```python
from build123d import *

# Parameters (mm, degrees)
SKETCH1_W                = 16
SKETCH1_H                = 24
SKETCH1_R                = 2.25
BOSS_EXTRUDE1_DEPTH      = 5
BOSS_EXTRUDE2_DEPTH      = 17
BOSS_EXTRUDE2_DEPTH_BACK = 5
SKETCH2_W                = 4
SKETCH2_H                = 24
SKETCH3_R                = 3.75
CUT_EXTRUDE1_DEPTH       = 30.732137495
BOSS_EXTRUDE3_DEPTH      = 2
FILLET1_R                = 3
SKETCH5_R                = 4
CUT_EXTRUDE2_DEPTH       = 2


with BuildPart() as part:
    # Sketch1 → Boss-Extrude1 (new body)
    with BuildSketch(Plane.XY):
        Rectangle(SKETCH1_W, SKETCH1_H)
        with Locations((-2, 6)):
            Circle(SKETCH1_R, mode=Mode.SUBTRACT)
        with Locations((-2, -6)):
            Circle(SKETCH1_R, mode=Mode.SUBTRACT)
    extrude(amount=BOSS_EXTRUDE1_DEPTH)

    # Sketch2 → Boss-Extrude2 (add, two sides: drawn at the far end of the back side and taken through both)
    with BuildSketch(Plane.XY.offset(5).offset(-BOSS_EXTRUDE2_DEPTH_BACK)):
        with Locations((6, 0)):
            Rectangle(SKETCH2_W, SKETCH2_H)
    extrude(amount=BOSS_EXTRUDE2_DEPTH + BOSS_EXTRUDE2_DEPTH_BACK)

    # Sketch3 → Cut-Extrude1 (cut, through all)
    with BuildSketch(Plane(origin=(8, 0, 0), x_dir=(0, 0, -1), z_dir=(1, 0, 0))):
        with Locations(Location((-14, 0, 0), (0, 0, 90))):
            Circle(SKETCH3_R)
    extrude(amount=-CUT_EXTRUDE1_DEPTH, mode=Mode.SUBTRACT)

    # Sketch4 → Boss-Extrude3 (add)
    with BuildSketch(Plane.XZ.offset(12)):
        Polygon((4, 22), (-8, 5), (4, 5), align=None)
    extrude(amount=-BOSS_EXTRUDE3_DEPTH)

    # Fillet1
    # the kernel refuses this fillet: 3 mm, written as the material it takes off along each edge
    with BuildSketch(Plane(origin=(15.5, -12, 22), x_dir=(0, 1, 0), z_dir=(-1, 0, 0))) as fillet1_piece_1:
        with BuildLine():
            CenterArc((FILLET1_R, FILLET1_R), FILLET1_R, 180, 90)
            Line((0, FILLET1_R), (0, 0))
            Line((0, 0), (FILLET1_R, 0))
        make_face()
    extrude(amount=19, mode=Mode.SUBTRACT)
    with BuildSketch(Plane(origin=(-3.5, 12, 22), x_dir=(0, 0, -1), z_dir=(1, 0, 0))) as fillet1_piece_2:
        with BuildLine():
            CenterArc((FILLET1_R, -FILLET1_R), FILLET1_R, 90, 90)
            Line((0, -FILLET1_R), (0, 0))
            Line((0, 0), (FILLET1_R, 0))
        make_face()
    extrude(amount=19, mode=Mode.SUBTRACT)
    with BuildSketch(Plane(origin=(15.5, -12, 0), x_dir=(0, 1, 0), z_dir=(-1, 0, 0)), Plane(origin=(15.5, 12, 0), x_dir=(0, 0, 1), z_dir=(-1, 0, 0))) as fillet1_piece_3:
        with BuildLine():
            CenterArc((FILLET1_R, -FILLET1_R), FILLET1_R, 90, 90)
            Line((0, -FILLET1_R), (0, 0))
            Line((0, 0), (FILLET1_R, 0))
        make_face()
    extrude(amount=31, mode=Mode.SUBTRACT)

    # Sketch5 → Cut-Extrude2 (cut)
    with BuildSketch(Plane.XY.offset(5)):
        with Locations((-2, 6)):
            Circle(SKETCH5_R)
        with Locations((-2, -6)):
            Circle(SKETCH5_R)
    extrude(amount=-CUT_EXTRUDE2_DEPTH, mode=Mode.SUBTRACT)


solid = part.part
```
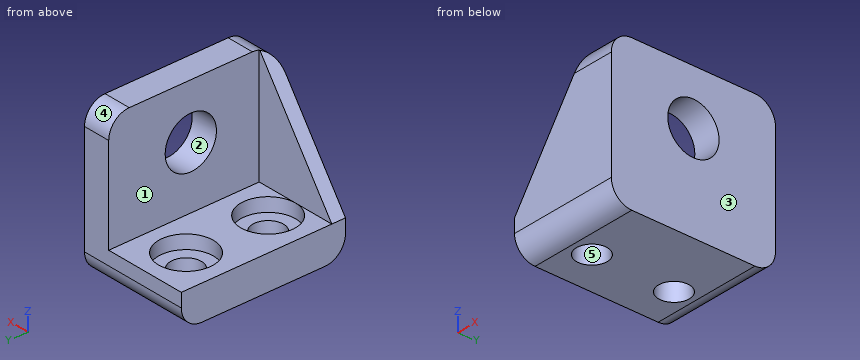
Geometry: final body of the model. Coordinates: model frame, mm. Face numbers are marked on the shaded views. A direction names the side the tool comes from. Coordinates: 2 decimals unless noted, no trailing zeros. Loops run counter-clockwise (first coordinate to the right, second up) from the corner with the lowest first, then second, coordinate; pieces in that order, holes last. Notation, with made-up numbers: M 42.25,52.5 L 71.25,52.5 A17 cw 71.25,60.5 Z; hole C 48.25,13 d8. An arc over 180 degrees is marked long. Put each result on its own line as item: value.
(1) Cut plane B-B on x = 5.75. Return the cut outline in (y, z).
Answer sheet:
outline: M -12,3 A3 ccw -9,0 L 9,0 A3 ccw 12,3 L 12,19 A3 ccw 9,22 L -9,22 A3 ccw -12,19 Z; hole C 0,14 d7.5
(2) First-contact query: pin 1 (4 mm diameter, centred on x = -3, y = -6.5, fed in from +Z); pin 2 (5 mm diameter, centred on x = -2.5, z = 16, fed in from +Y); pin 3 (10 mm diameter, centred on y = 0, z = 14, fed in from -X); pin 4 (1.5 mm diameter, centred on y = -1.5, z = 14.5, fed in from -X). Flat tips, straight axial feed; report the tip coordinate or a pass-through.
Answer sheet:
pin 1: stops at z = 3
pin 2: stops at y = -10
pin 3: stops at x = 4
pin 4: passes through
(3) Cut plane C-C on z = 12.75. Return the cut outline in (x, y), then the cut area to 3 significant figures.
Answer sheet:
outline: M -2.53,-12 L 8,-12 L 8,-3.54 L 4,-3.54 L 4,-10 L -2.53,-10 Z; M 4,3.54 L 8,3.54 L 8,12 L 4,12 Z
area: 80.8 mm^2
(4) Material intervals for probe 1 along Y at (x, z) = (-2, 4.45); probe 2 along X at (y, z) = (6, 1.15); probe 3 along Y at (x, z) = (-2, 2.2), sorted ascending.
Answer sheet:
probe 1: y = -12 to -10, -2 to 2, 10 to 12
probe 2: x = -8 to -4.25, 0.25 to 8
probe 3: y = -11.89 to -8.25, -3.75 to 3.75, 8.25 to 11.89
(5) Access query for the marked faces 1 and 2. Directions: +Z, -Z, +X, -X, +Y, -Y. A direction counts if a zero-diameter tool reaches every point of the face in a straight line with its end or side. Return the directions, or none.
Answer sheet:
face 1: +Z, -X, +Y
face 2: +X, -X
(6) Draft query along X for the marked faces 3, 4 and 5. Return one class per face: pulls with the +X half, pulls with the -X half, needs draft (parallel to the pull), parting line crosses it, or undercut.
Answer sheet:
face 3: pulls with the +X half
face 4: needs draft
face 5: undercut
(7) Cut plane A-A on y = 0. Return the cut outline in (x, z), then the cut area to 3 significant figures.
Answer sheet:
outline: M -8,0 L 8,0 L 8,10.25 L 4,10.25 L 4,5 L -8,5 Z; M 4,17.75 L 8,17.75 L 8,22 L 4,22 Z
area: 118 mm^2
(8) Cut plane D-D on y = 6. Return the cut outline in (x, z), then the cut area to 4 significant figures.
Answer sheet:
outline: M -8,0 L -4.25,0 L -4.25,3 L -6,3 L -6,5 L -8,5 Z; M 0.25,0 L 8,0 L 8,22 L 4,22 L 4,5 L 2,5 L 2,3 L 0.25,3 Z
area: 118.5 mm^2
